Source: three-view drawing plus pictorial views. Frame: mm from the lowest corner of the part. A direction names the side the tool comes from. Round coordinates to 2 decimals unless told otherwise and drop trailing zeros. Order: outer loops, then holes, each group sorted by start corner. A loop starts at its lowest first (then second) coordinate and runs counter-clockwise, first axis right, second up. Notation, with made-up numbers: (-20.75, -14) -> (2.25, -14) arc R22 ccw to (2.25, -3) -> close; hole circle Ø8 at (2, 89.5). An arc over 180 degrees is marked (long way). Use a Markdown table: item, result.
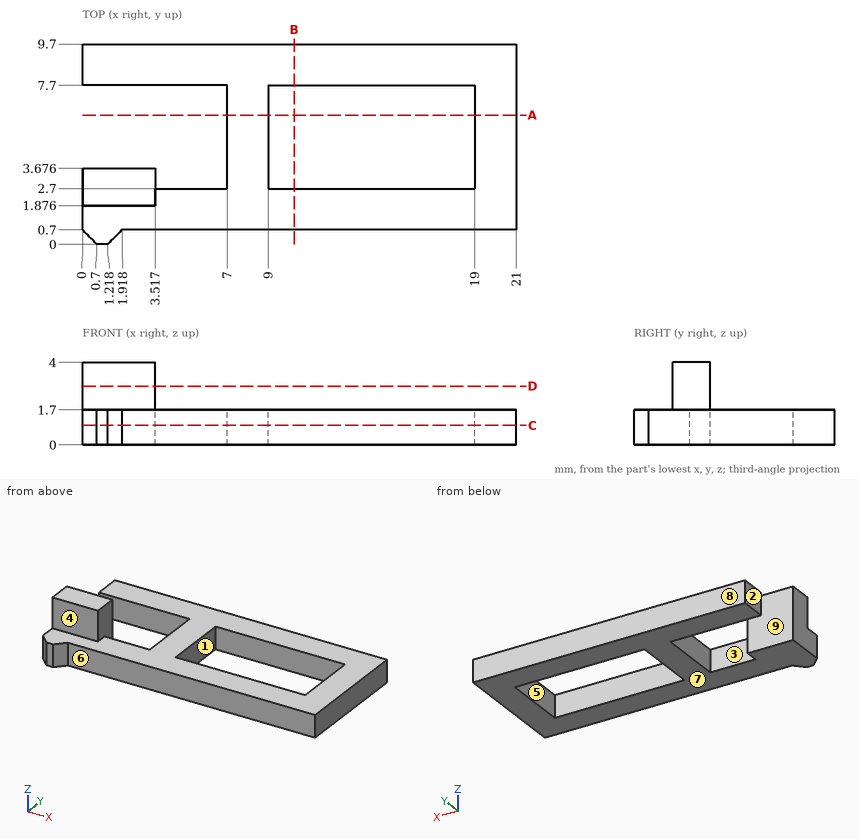
1) Set-up query: the marked faces 5, 6, 7, 8 and 9. Return all of +Z, -Z, +X, -X, +Y, -Y with unobstructed straight access to the full face (end or side cutting, diameter ignored); none if empty.
Results found:
| item | result |
|---|---|
| face 5 | +Z, -Z |
| face 6 | +Z, -Z, +X, -Y |
| face 7 | -Z, +X, -X, +Y, -Y |
| face 8 | +Z, -Z, +X, -X, +Y |
| face 9 | +Z, -Z, -X |
2) Cut plane A-A on y = 6.25. Return loops of the section in (x, z).
Results found:
| item | result |
|---|---|
| outline | (7, 0) -> (9, 0) -> (9, 1.7) -> (7, 1.7) -> close; (19, 0) -> (21, 0) -> (21, 1.7) -> (19, 1.7) -> close |
3) Pin query (flat end, axial travel): pin 1 Ø1 at (x, z) = (6.5, 0.5) entering from -Y; pin 2 Ø3 at (x, y) = (12, 5.5) entering from +Z; pin 3 Ø1 at (y, z) = (4.5, 0.5) entering from -X; pin 4 Ø0.9 at (y, z) = (2.5, 3) entering from +X. Return the tip coordinate at first contact, or that it passes through.
Results found:
| item | result |
|---|---|
| pin 1 | stops at y = 0.7 |
| pin 2 | passes through |
| pin 3 | stops at x = 7 |
| pin 4 | stops at x = 3.52 |
4) Cut plane B-B on x = 10.25. Return loops of the section in (y, z).
Results found:
| item | result |
|---|---|
| outline | (0.7, 0) -> (2.7, 0) -> (2.7, 1.7) -> (0.7, 1.7) -> close; (7.7, 0) -> (9.7, 0) -> (9.7, 1.7) -> (7.7, 1.7) -> close |
5) Cut plane C-C on z = 0.95. Return loops of the section in (x, y), and give its area (3 significant figures).
Results found:
| item | result |
|---|---|
| outline | (0, 0.7) -> (0.7, 0) -> (1.22, 0) -> (1.92, 0.7) -> (21, 0.7) -> (21, 9.7) -> (0, 9.7) -> (0, 7.7) -> (7, 7.7) -> (7, 2.7) -> (3.52, 2.7) -> (3.52, 3.68) -> (0, 3.68) -> close; hole (9, 2.7) -> (19, 2.7) -> (19, 7.7) -> (9, 7.7) -> close |
| area | 108 mm² |
6) Pull-direction query (X, two-part tool) for the marked faces 1, 2, 3 and 4; classes: +X half, -X half, draft (parallel to the pull), parting line (faces both ways), or undercut.
Results found:
| item | result |
|---|---|
| face 1 | undercut |
| face 2 | -X half |
| face 3 | undercut |
| face 4 | draft |
7) Cut plane D-D on z = 2.85. Return loops of the section in (x, y).
Results found:
| item | result |
|---|---|
| outline | (0, 1.88) -> (3.52, 1.88) -> (3.52, 3.68) -> (0, 3.68) -> close |
8) Line query: L1, parallel to X at y = 3.5, z = 0.85; L2, parallel to X at y = 6.5, z = 0.2; L3, parallel to Y at x = 15.5, z = 0.5. Output: solid intervals per line, ascending. Write a range as [from, to].
Results found:
| item | result |
|---|---|
| L1 | x = [0, 3.52], [7, 9], [19, 21] |
| L2 | x = [7, 9], [19, 21] |
| L3 | y = [0.7, 2.7], [7.7, 9.7] |
